For this review, take the finished solid that the model builds, in its own axes (mm). Face numbers are marked on the shaded views. A direction names the side the tool comes from. Give positions to 0.01 mm unless a question says otherwise; leave off trailing zeros. Write each loop counter-clockwise with the first axis right and the second up, starting at its lowest first coordinate (ties: lowest second). Pieces come first, ordered by that corner, then holes.
1) We need section D-D on x = 9. Give the boundary of the cut face in (y, z).
2) We need section A-A on x = -0.75. Give the boundary of the cut face in (y, z), and give its area (3 significant figures).
3) We need section C-C on y = 4.5. Give the number of separate pieces and of enclosed holes in the cut face, and give its area (4 significant figures).
4) Draft analysis for pull direction X (two halves, no side actions). For the marked faces 3, 4 and 5, state which applies: pulls with the +X half, pulls with the -X half, needs draft (parallel to the pull), parting line crosses it, or undercut.
5) Machinability: for the marked faces 1 and 2, which of the approach directions +Z, -Z, +X, -X, +Y, -Y give a long, thin tool a straight path to every point of the face, cutting with its end or side? Answer none if there is none.
6) Wall thickness on line 1 along Z through (x, y) = (2.5, 4); line 2 along Z through (x, y) = (-6.25, 5); line 3 along X through (y, z) = (3.75, -0.5): over which ranges is each line inside the solid? List them lowest first.
7) We need section B-B on z = 2. Give the boundary of the cut face in (x, y).
from build123d import *

# Parameters (mm, degrees)
SKETCH1_W           = 22.5
SKETCH1_H           = 7
BASE_DEPTH          = 2.5
RIMS_DEPTH          = 4
CHAMFER1_SIZE       = 0.5
SKETCH3_W           = 0.3
SKETCH3_H           = 0.3
BOSS_EXTRUDE3_DEPTH = 3.5


with BuildPart() as part:
    # Sketch1 → Base (new body)
    with BuildSketch(Plane(origin=(0, 0, 0), x_dir=(1, 0, 0), z_dir=(0, 1, 0))):
        Rectangle(SKETCH1_W, SKETCH1_H)
    extrude(amount=BASE_DEPTH)

    # Sketch2 → rims (add)
    with BuildSketch(Plane(origin=(0, 2.5, 0), x_dir=(1, 0, 0), z_dir=(0, 1, 0))):
        Polygon((-1.25, -2.5), (-1.25, -3.5), (-11.25, -3.5), (-11.25, 3.5), (11.25, 3.5), (11.25, -3.5), (1.25, -3.5), (1.25, -2.5), (10.25, -2.5), (10.25, 2.5), (-10.25, 2.5), (-10.25, -2.5), align=None)
    extrude(amount=RIMS_DEPTH)

    # Chamfer1
    chamfer1_edges = [part.edges().sort_by_distance(p)[0] for p in [
        (-5.75, 6.5, 2.5),
        (-10.25, 6.5, 0),
        (0, 6.5, -2.5),
        (10.25, 6.5, 0),
        (5.75, 6.5, 2.5),
    ]]
    chamfer(chamfer1_edges, length=CHAMFER1_SIZE)

    # Sketch3 → Boss-Extrude3 (add)
    with BuildSketch(Plane(origin=(0, 2.5, 0), x_dir=(1, 0, 0), z_dir=(0, 1, 0))):
        with Locations((-8.6, -0.85)):
            Rectangle(SKETCH3_W, SKETCH3_H)
        with Locations((-8.6, 0.85)):
            Rectangle(SKETCH3_W, SKETCH3_H)
        with Locations((-7.2, -0.85)):
            Rectangle(SKETCH3_W, SKETCH3_H)
        with Locations((-5.8, -0.85)):
            Rectangle(SKETCH3_W, SKETCH3_H)
        with Locations((-4.4, -0.85)):
            Rectangle(SKETCH3_W, SKETCH3_H)
        with Locations((-3, -0.85)):
            Rectangle(SKETCH3_W, SKETCH3_H)
        with Locations((-1.6, -0.85)):
            Rectangle(SKETCH3_W, SKETCH3_H)
        with Locations((-0.2, -0.85)):
            Rectangle(SKETCH3_W, SKETCH3_H)
        with Locations((1.2, -0.85)):
            Rectangle(SKETCH3_W, SKETCH3_H)
        with Locations((2.6, -0.85)):
            Rectangle(SKETCH3_W, SKETCH3_H)
        with Locations((4, -0.85)):
            Rectangle(SKETCH3_W, SKETCH3_H)
        with Locations((5.4, -0.85)):
            Rectangle(SKETCH3_W, SKETCH3_H)
        with Locations((6.8, -0.85)):
            Rectangle(SKETCH3_W, SKETCH3_H)
        with Locations((8.2, -0.85)):
            Rectangle(SKETCH3_W, SKETCH3_H)
        with Locations((-7.2, 0.85)):
            Rectangle(SKETCH3_W, SKETCH3_H)
        with Locations((-5.8, 0.85)):
            Rectangle(SKETCH3_W, SKETCH3_H)
        with Locations((-4.4, 0.85)):
            Rectangle(SKETCH3_W, SKETCH3_H)
        with Locations((-3, 0.85)):
            Rectangle(SKETCH3_W, SKETCH3_H)
        with Locations((-1.6, 0.85)):
            Rectangle(SKETCH3_W, SKETCH3_H)
        with Locations((-0.2, 0.85)):
            Rectangle(SKETCH3_W, SKETCH3_H)
        with Locations((1.2, 0.85)):
            Rectangle(SKETCH3_W, SKETCH3_H)
        with Locations((2.6, 0.85)):
            Rectangle(SKETCH3_W, SKETCH3_H)
        with Locations((4, 0.85)):
            Rectangle(SKETCH3_W, SKETCH3_H)
        with Locations((5.4, 0.85)):
            Rectangle(SKETCH3_W, SKETCH3_H)
        with Locations((6.8, 0.85)):
            Rectangle(SKETCH3_W, SKETCH3_H)
    extrude(amount=BOSS_EXTRUDE3_DEPTH)


solid = part.part
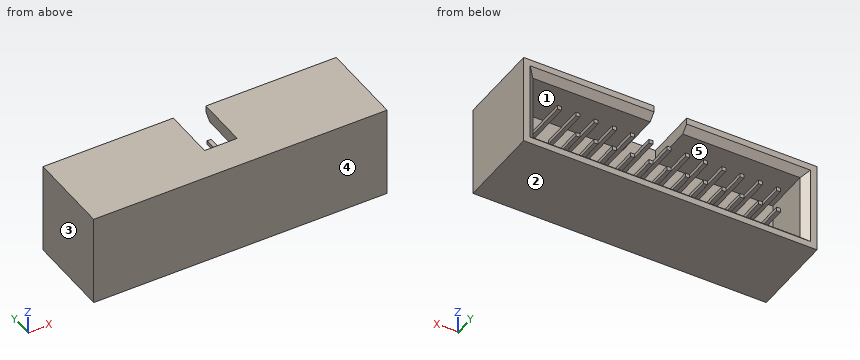
Results list:
1. outline: (0, -3.5) - (6.5, -3.5) - (6.5, -3) - (6, -2.5) - (2.5, -2.5) - (2.5, 2.5) - (6, 2.5) - (6.5, 3) - (6.5, 3.5) - (0, 3.5) - close
2. outline: (0, -3.5) - (6.5, -3.5) - (6.5, -3) - (6, -2.5) - (2.5, -2.5) - (2.5, 3.5) - (0, 3.5) - close
2. area: 21.4 mm2
3. separate pieces: 26
3. enclosed holes: 0
3. area: 54.75 mm2
4. face 3: pulls with the -X half
4. face 4: needs draft
4. face 5: undercut
5. face 1: +Y
5. face 2: -Z, +X, -X, +Y, -Y
6. line 1: z = -3.5 to -2.5, -1 to -0.7, 0.7 to 1, 2.5 to 3.5
6. line 2: z = -3.5 to -2.5, 2.5 to 3.5
6. line 3: x = -11.25 to -10.25, 10.25 to 11.25
7. outline: (-11.25, 0) - (11.25, 0) - (11.25, 6.5) - (10.75, 6.5) - (10.25, 6) - (10.25, 2.5) - (-10.25, 2.5) - (-10.25, 6) - (-10.75, 6.5) - (-11.25, 6.5) - close
